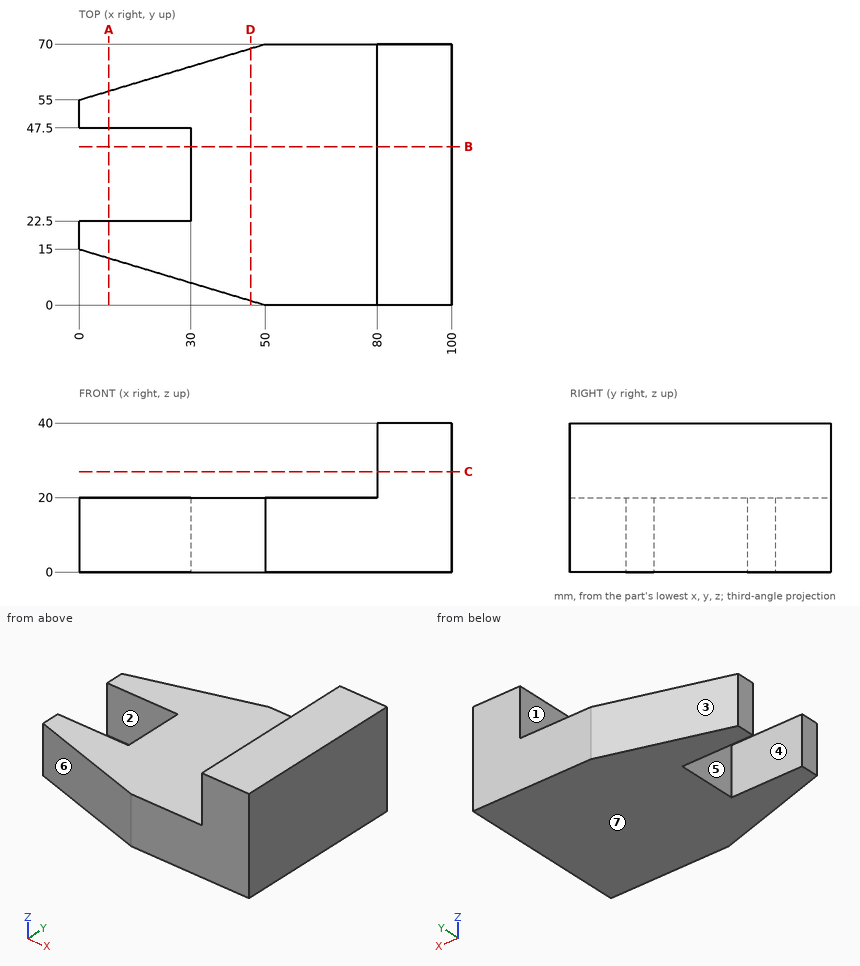
Geometry check sheet. Reference: drawing and pictorial views, mm from the part's lowest x, y, z. A direction names the side the tool comes from. Give positions to 0.01 mm unless a question says otherwise; leave off trailing zeros. Order: outer loops, then holes, each group sorted by start corner. A loop starts at its lowest first (then second) coordinate and runs counter-clockwise, first axis right, second up. Notation, with made-up numbers: M -2.75,62.25 L 30.25,62.25 A20 ccw 30.25,80.25 Z; hole C 47.25,-31 d10. An arc over 180 degrees is marked long. Answer in a Markdown table with one row per item.
1) Cross-section at B-B, the plane y = 42.5. Enter the section's corners in (x, z), plus the area to 3 significant figures.
Filled sheet:
| item | result |
|---|---|
| outline | M 30,0 L 100,0 L 100,40 L 80,40 L 80,20 L 30,20 Z |
| area | 1,800 mm2 |
2) Release check for a two-part mould opening along Y. For the marked faces 4, 5, 6 and 7 record: +Y half, -Y half, draft (parallel to the pull), parting line (faces both ways), or undercut.
Filled sheet:
| item | result |
|---|---|
| face 4 | undercut |
| face 5 | undercut |
| face 6 | -Y half |
| face 7 | draft |
3) Cross-section at D-D, the plane x = 46. Enter the section's corners in (y, z), plus the area to 3 significant figures.
Filled sheet:
| item | result |
|---|---|
| outline | M 1.2,0 L 68.8,0 L 68.8,20 L 1.2,20 Z |
| area | 1,350 mm2 |
4) Cross-section at C-C, the plane z = 27. Enter the section's corners in (x, y), plus the area to 3 significant figures.
Filled sheet:
| item | result |
|---|---|
| outline | M 80,0 L 100,0 L 100,70 L 80,70 Z |
| area | 1,400 mm2 |
5) Cross-section at A-A, the plane x = 8. Enter the section's corners in (y, z).
Filled sheet:
| item | result |
|---|---|
| outline | M 12.6,0 L 22.5,0 L 22.5,20 L 12.6,20 Z; M 47.5,0 L 57.4,0 L 57.4,20 L 47.5,20 Z |
6) Access from +Z, -Z, +X, -X, +Y, -Y to the whole of each face (thin tool, end or side, straight path). Record for the marked faces 1, 2 and 3.
Filled sheet:
| item | result |
|---|---|
| face 1 | +Z, -X, +Y, -Y |
| face 2 | +Z, -Z, -X |
| face 3 | +Z, -Z, -X, +Y |
7) Thickness scan on L1, parallel to Z at x = 78, y = 32; L2, parallel to X at y = 33, z = 2; L3, parallel to X at y = 54, z = 27.5. Record the ranges inside material, lowest first. Write a range as [from, to].
Filled sheet:
| item | result |
|---|---|
| L1 | z = [0, 20] |
| L2 | x = [30, 100] |
| L3 | x = [80, 100] |
8) Gauge pin test, flat ends, axial feed: P1, Ø3, axis at x = 23, z = 19.5, coming from the -Y side; P2, Ø2, axis at y = 50.5, z = 25.5, coming from the -X side; P3, Ø4, axis at y = 31.5, z = 9.5, coming from the -X side. Record the tip position at first contact, or that the pin passes through.
Filled sheet:
| item | result |
|---|---|
| P1 | stops at y = 7.65 |
| P2 | stops at x = 80 |
| P3 | stops at x = 30 |
